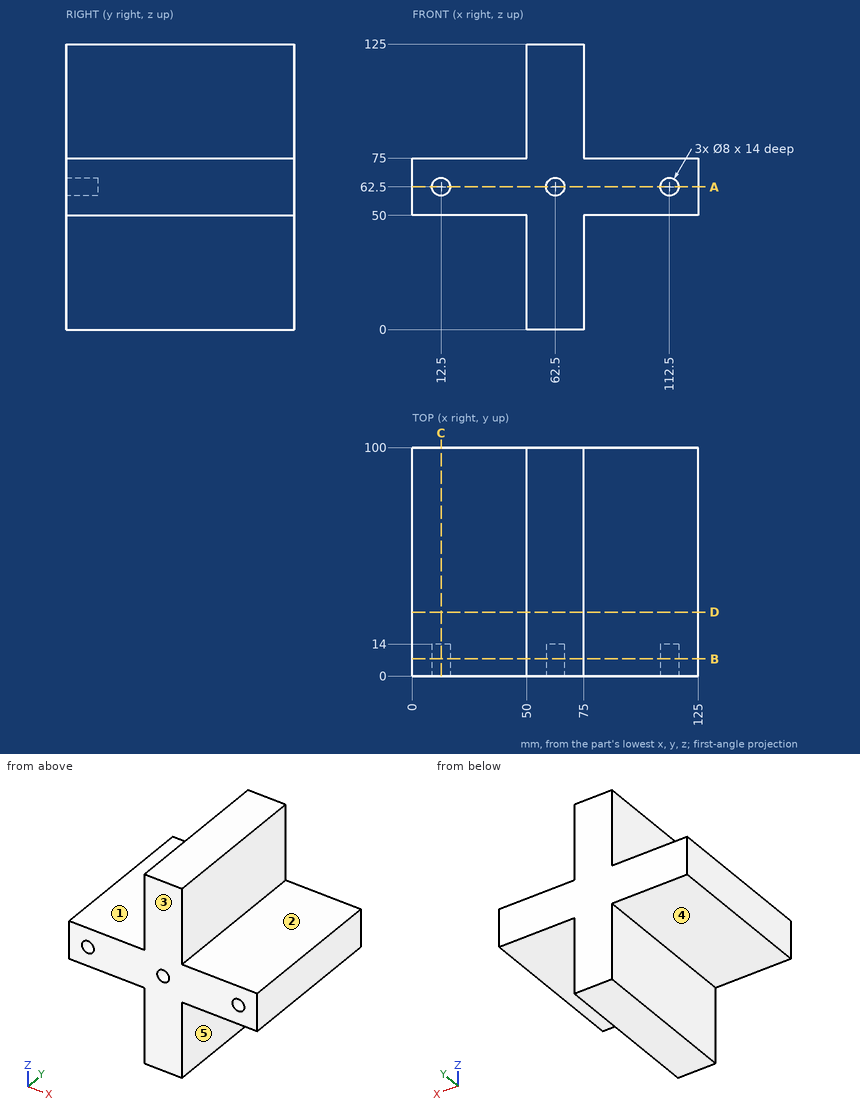
The drawing under review shows one solid part. Ordinate dimensions are in mm from its lowest x, y, z. A direction names the side the tool comes from. Give positions to 0.01 mm unless a question says otherwise; leave off trailing zeros. Write each loop counter-clockwise with the first axis right and the second up, starting at its lowest first coordinate (ties: lowest second). Pieces come first, ordered by that corner, then holes. Notation, with made-up numbers: (44, 3.25) -> (91, 3.25) arc R13 cw to (91, 11.25) -> close; hole circle Ø3 at (12.25, 49.5). An arc over 180 degrees is marked (long way). Answer in a Markdown table with one row per item.
(1) To check wall thickness, follow probe 1 along X at (y, z) = (4, 62); probe 2 along X at (y, z) = (89, 97); probe 3 along Z at (x, y) = (12, 10). State the ranges of each line that lie inside material, in increasing order.
Results:
| item | result |
|---|---|
| probe 1 | 0 to 8.53, 16.47 to 58.53, 66.47 to 108.53, 116.47 to 125 |
| probe 2 | 50 to 75 |
| probe 3 | 50 to 58.53, 66.47 to 75 |
(2) For the marked faces 1, 2, 3, 4 and 5, list the 3-axis set-ups (+Z, -Z, +X, -X, +Y, -Y) from which the entire face can be reached by the end or side of a thin tool; tool diameter is ignored.
Results:
| item | result |
|---|---|
| face 1 | +Z, -X, +Y, -Y |
| face 2 | +Z, +X, +Y, -Y |
| face 3 | +Z, -Z, +X, -X, -Y |
| face 4 | -Z, -X, +Y, -Y |
| face 5 | -Z, +X, +Y, -Y |
(3) Consider section D-D (y = 28). State the section outline as (x, z) points.
Results:
| item | result |
|---|---|
| outline | (0, 50) -> (50, 50) -> (50, 0) -> (75, 0) -> (75, 50) -> (125, 50) -> (125, 75) -> (75, 75) -> (75, 125) -> (50, 125) -> (50, 75) -> (0, 75) -> close |
(4) Consider section A-A (z = 62.5). State the section outline as (x, y) points.
Results:
| item | result |
|---|---|
| outline | (0, 0) -> (8.5, 0) -> (8.5, 14) -> (16.5, 14) -> (16.5, 0) -> (58.5, 0) -> (58.5, 14) -> (66.5, 14) -> (66.5, 0) -> (108.5, 0) -> (108.5, 14) -> (116.5, 14) -> (116.5, 0) -> (125, 0) -> (125, 100) -> (0, 100) -> close |
(5) Consider section C-C (x = 12.5). State the section outline as (y, z) points, then the cut area to 3 significant figures.
Results:
| item | result |
|---|---|
| outline | (0, 50) -> (100, 50) -> (100, 75) -> (0, 75) -> (0, 66.5) -> (14, 66.5) -> (14, 58.5) -> (0, 58.5) -> close |
| area | 2,390 mm2 |
(6) Clearance check with flat-ended pins moving along their axes: pin 1 (1.5 mm diameter, centred on x = 76, z = 48, fed in from +Y); pin 2 (9 mm diameter, centred on x = 12.5, z = 62.5, fed in from -Y); pin 3 (25 mm diameter, centred on y = 29.5, z = 23, fed in from +X); pin 4 (15 mm diameter, centred on x = 97, y = 64.5, fed in from -Z). State where each tip first meets the part, or that it passes through.
Results:
| item | result |
|---|---|
| pin 1 | through |
| pin 2 | y = 0 |
| pin 3 | x = 75 |
| pin 4 | z = 50 |
(7) Consider section B-B (y = 7.5). State the section outline as (x, z) points.
Results:
| item | result |
|---|---|
| outline | (0, 50) -> (50, 50) -> (50, 0) -> (75, 0) -> (75, 50) -> (125, 50) -> (125, 75) -> (75, 75) -> (75, 125) -> (50, 125) -> (50, 75) -> (0, 75) -> close; hole circle Ø8 at (12.5, 62.5); hole circle Ø8 at (62.5, 62.5); hole circle Ø8 at (112.5, 62.5) |
